Check sheet for the modelled part. Datum: model origin and axes. Units: mm. Face numbers are marked on the shaded views. Give positions to 0.01 mm unless a question says otherwise; leave off trailing zeros. Write each loop counter-clockwise with the first axis right and the second up, starting at its lowest first coordinate (ties: lowest second). Pieces come first, ordered by that corner, then holes. Notation, with made-up numbers: M -13,72 L 25,72 A30 ccw 25,111 Z; hole C 36.25,13.25 d6. An arc over 180 degrees is marked long. Write item = value, one per line. Start each with the question number.
1) Sectioned sample at B-B, the plane y = 0. Record the cut outline in (x, z).
2) Scan lines: L1, parallel to X at y = 14, z = 0; L2, parallel to X at y = -13.45, z = 0; L3, parallel to Z at x = 205, y = 13. Record each from-to range of solid material in increasing order.
3) Draft check along Z on the marked faces 1 and 2. Enter one of: pulls with the +Z half, pulls with the -Z half, needs draft (parallel to the pull), parting line crosses it, or undercut.
4) Sectioned sample at C-C, the plane x = 205. Record the cut outline in (y, z), then the cut area to 3 significant figures.
5) Sectioned sample at D-D, the plane x = 4. Record the cut outline in (y, z), then the cut area to 3 significant figures.
6) Gauge pin test, flat ends, axial feed: pin 1 (8 mm diameter, centred on x = 123, y = -4, fed in from +Z); pin 2 (3 mm diameter, centred on y = 7, z = 0.5, fed in from +X); pin 3 (2.5 mm diameter, centred on x = 155.5, y = 12, fed in from -Z); pin 4 (2 mm diameter, centred on y = -9, z = -5.5, fed in from +X). Record the tip position at first contact, or that the pin passes through.
7) Sectioned sample at A-A, the plane z = 0. Record the cut outline in (x, y), then the cut area to 3 significant figures.
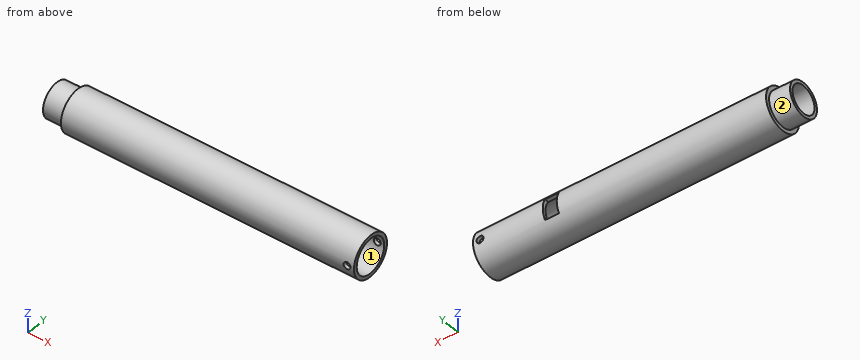
from build123d import *

# Parameters (mm, degrees)
ESBO_O1_R                  = 15
ESBO_O1_R_2                = 12.5
RESSALTO_EXTRUS_O1_DEPTH   = 210
RESSALTO_EXTRUS_O3_START   = 15
ESBO_O2_R                  = 12.25
ESBO_O2_R_2                = 10
RESSALTO_EXTRUS_O3_DEPTH   = 15
CORTE_EXTRUS_O2_DEPTH      = 300
CORTE_EXTRUS_O2_DEPTH_BACK = 300
ESBO_O4_R                  = 2.5
ESBO_O6_W                  = 10
ESBO_O6_H                  = 15
CORTE_EXTRUS_O4_DEPTH      = 20
ESBO_O7_R                  = 12.5
RESSALTO_EXTRUS_O4_DEPTH   = 10
ESBO_O11_R                 = 10
CORTE_EXTRUS_O8_DEPTH      = 20


with BuildPart() as part:
    # Esbo_o1 → Ressalto-extrus_o1 (new body)
    with BuildSketch(Plane(origin=(0, 0, 0), x_dir=(0, 0, -1), z_dir=(1, 0, 0))):
        Circle(ESBO_O1_R)
        Circle(ESBO_O1_R_2, mode=Mode.SUBTRACT)
    extrude(amount=RESSALTO_EXTRUS_O1_DEPTH)

    # Esbo_o4 → Corte-extrus_o2 (cut, two sides: drawn at the far end of the back side and taken through both)
    with BuildSketch(Plane(origin=(0, 0, 0), x_dir=(1, 0, 0), z_dir=(0, 1, 0)).offset(-CORTE_EXTRUS_O2_DEPTH_BACK)):
        with Locations(Location((205, 0, 0), (0, 0, 90))):
            Circle(ESBO_O4_R)
    extrude(amount=CORTE_EXTRUS_O2_DEPTH + CORTE_EXTRUS_O2_DEPTH_BACK, mode=Mode.SUBTRACT)

    # Esbo_o6 → Corte-extrus_o4 (cut)
    with BuildSketch(Plane(origin=(0, 0, 0), x_dir=(1, 0, 0), z_dir=(0, 1, 0))):
        with Locations((155, 0)):
            Rectangle(ESBO_O6_W, ESBO_O6_H)
    extrude(amount=CORTE_EXTRUS_O4_DEPTH, mode=Mode.SUBTRACT)



with BuildPart() as body_2:
    # Esbo_o2 → Ressalto-extrus_o3 (new body)
    with BuildSketch(Plane.ZY.offset(RESSALTO_EXTRUS_O3_START)):
        Circle(ESBO_O2_R)
        Circle(ESBO_O2_R_2, mode=Mode.SUBTRACT)
    extrude(amount=-RESSALTO_EXTRUS_O3_DEPTH)


with BuildPart() as part_1:
    add(part.part)

    add(body_2.part)  # Ressalto-extrus_o4 merges body 2
    # Esbo_o7 → Ressalto-extrus_o4 (add)
    with BuildSketch(Plane.ZY):
        Circle(ESBO_O7_R)
    extrude(amount=-RESSALTO_EXTRUS_O4_DEPTH)

    # Esbo_o11 → Corte-extrus_o8 (cut)
    with BuildSketch(Plane.ZY):
        Circle(ESBO_O11_R)
    extrude(amount=-CORTE_EXTRUS_O8_DEPTH, mode=Mode.SUBTRACT)


solid = part_1.part
Data:
q1.outline = M -15,-12.25 L 0,-12.25 L 0,-15 L 210,-15 L 210,-12.5 L 10,-12.5 L 10,-10 L -15,-10 Z; M -15,10 L 10,10 L 10,12.5 L 210,12.5 L 210,15 L 0,15 L 0,12.25 L -15,12.25 Z
q2.L1 = 0 to 150, 160 to 202.5, 207.5 to 210
q2.L2 = 0 to 202.5, 207.5 to 210
q2.L3 = -7.48 to -2.5, 2.5 to 7.48
q3.face_1 = undercut
q3.face_2 = parting line crosses it
q4.outline = M -14.79,-2.5 A15 ccw 14.79,-2.5 L 12.25,-2.5 A12.5 cw -12.25,-2.5 Z; M -14.79,2.5 L -12.25,2.5 A12.5 cw 12.25,2.5 L 14.79,2.5 A15 ccw Z
q4.area = 191 mm2
q5.outline = C 0,0 d30; hole C 0,0 d20
q5.area = 393 mm2
q6.pin_1 = 15
q6.pin_2 = through
q6.pin_3 = -10.46
q6.pin_4 = 10
q7.outline = M -15,-12.25 L 0,-12.25 L 0,-15 L 202.5,-15 L 202.5,-12.5 L 10,-12.5 L 10,-10 L -15,-10 Z; M -15,10 L 10,10 L 10,12.5 L 150,12.5 L 150,15 L 0,15 L 0,12.25 L -15,12.25 Z; M 160,12.5 L 202.5,12.5 L 202.5,15 L 160,15 Z; M 207.5,-15 L 210,-15 L 210,-12.5 L 207.5,-12.5 Z; M 207.5,12.5 L 210,12.5 L 210,15 L 207.5,15 Z
q7.area = 1,120 mm2
